Input: part model. Units: mm. Frame: model coordinates. Face numbers are marked on the shaded views. A direction names the side the tool comes from. Give positions to 0.01 mm unless a question says otherwise; leave off trailing zeros. Loops run counter-clockwise (first coordinate to the right, second up) from the corner with the lowest first, then second, coordinate; pieces in that order, holes last. Notation, with made-up numbers: (-14.5, 76) - (41.5, 76) arc R10 ccw to (41.5, 90) - close; hole circle Ø1 at (10, -27). An arc over 180 degrees is marked (long way). Answer as a JSON object with one key per item and string values.
from build123d import *

# Parameters (mm, degrees)
BOSS_EXTRUDE1_DEPTH      = 15.875
BOSS_EXTRUDE1_DEPTH_BACK = 46.0375
SKETCH1_R                = 3.175
REVOLVE1_ANGLE           = 180
CUT_EXTRUDE1_DEPTH       = 8.382
CUT_EXTRUDE1_DEPTH_BACK  = 9.398
SKETCH3_W                = 2.54
SKETCH3_H                = 12.7
SKETCH4_W                = 2.54
SKETCH4_H                = 12.81199514
CUT_EXTRUDE2_DEPTH       = 1.524


with BuildPart() as part:
    # Sketch1 → Boss-Extrude1 (new, two sides: drawn at the far end of the back side and taken through both)
    with BuildSketch(Plane.XY.offset(-BOSS_EXTRUDE1_DEPTH_BACK)):
        Circle(SKETCH1_R)
    extrude(amount=BOSS_EXTRUDE1_DEPTH + BOSS_EXTRUDE1_DEPTH_BACK)

    # Sketch2 → Revolve1 (revolve)
    with BuildSketch(Plane.XY.offset(15.875)):
        with BuildLine():
            Line((0, -4.7625), (0, 4.7625))
            ThreePointArc((0, 4.7625), (4.7625, 0), (0, -4.7625))
        make_face()
    revolve(axis=Axis((0, -4.7625, 15.875), (0, -1, 0)), revolution_arc=REVOLVE1_ANGLE)

    # Sketch3 → Cut-Extrude1 (cut, two sides: drawn at the far end of the back side and taken through both)
    with BuildSketch(Plane(origin=(2.54, 0, 0), x_dir=(0, 0, -1), z_dir=(1, 0, 0)).offset(-CUT_EXTRUDE1_DEPTH_BACK)):
        with Locations((-20.955, -1.5875)):
            Rectangle(SKETCH3_W, SKETCH3_H)
    extrude(amount=CUT_EXTRUDE1_DEPTH + CUT_EXTRUDE1_DEPTH_BACK, mode=Mode.SUBTRACT)

    # Sketch4 → Cut-Extrude2 (cut)
    with BuildSketch(Plane.XY.offset(19.685)):
        with Locations((0, -0.792879604)):
            Rectangle(SKETCH4_W, SKETCH4_H)
    extrude(amount=-CUT_EXTRUDE2_DEPTH, mode=Mode.SUBTRACT)


solid = part.part
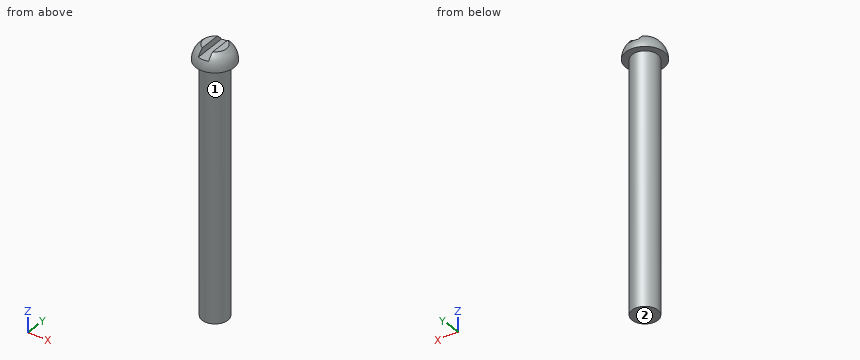
Item 1: Cut plane A-A (x = 0). Return loops of the section in (y, z) (1 decimal), then the cut area to 3 significant figures.
Geometry check:
{"outline": "(-4.8, 15.9) - (-3.2, 15.9) - (-3.2, -46) - (3.2, -46) - (3.2, 15.9) - (4.8, 15.9) arc R4.8 ccw to (4.2, 18.2) - (-4.2, 18.2) arc R4.8 ccw to start", "area": "414 mm2"}
Item 2: Cut plane D-D (x = 4). Return loops of the section in (y, z) (3 decimals), then the cut area to 3 significant figures.
Geometry check:
{"outline": "(-2.585, 15.875) - (2.585, 15.875) arc R2.585 ccw to start", "area": "10.5 mm2"}
Item 3: Access query for the marked faces 1 and 2. Directions: +Z, -Z, +X, -X, +Y, -Y. A direction counts if a zero-diameter tool reaches every point of the face in a straight line with its end or side. Return the directions, or none.
Geometry check:
{"face 1": "-Z", "face 2": "-Z, +X, -X, +Y, -Y"}
Item 4: Cut plane C-C (z = -5.5). Return loops of the section in (x, y) (3 decimals).
Geometry check:
{"outline": "circle Ø6.35 at (0, 0)"}
Item 5: Cut plane B-B (y = 0). Return loops of the section in (x, z) (1 decimal).
Geometry check:
{"outline": "(-4.8, 15.9) - (-3.2, 15.9) - (-3.2, -46) - (3.2, -46) - (3.2, 15.9) - (4.8, 15.9) arc R4.8 ccw to (2.9, 19.7) - (1.3, 19.7) - (1.3, 18.2) - (-1.3, 18.2) - (-1.3, 19.7) - (-2.9, 19.7) arc R4.8 ccw to start"}
Item 6: Material intervals for line 1 (Z direction, x = 1, y = 1); line 2 (Y direction, x = -0.25, z = 11.5); line 3 (Y direction, x = 0.5, z = -3), sorted ascending. Write a range as [from, to].
Geometry check:
{"line 1": "z = [-46.04, 18.16]", "line 2": "y = [-3.17, 3.17]", "line 3": "y = [-3.14, 3.14]"}
Item 7: Contact query for flat-ended pins moving along their axis: P1, Ø5, axis at y = 2.5, z = -34.5, coming from the +X side (3 decimals); P2, Ø1.5, axis at y = 1.5, z = 1.5, coming from the -X side; P3, Ø4, axis at x = 1, z = -23.5, coming from the +Y side (3 decimals). Output: stop coordinate, or through.
Geometry check:
{"P1": "stops at x = 3.175", "P2": "stops at x = -3.09", "P3": "stops at y = 3.175"}
